For this review, use the dimensioned drawing (mm, ordinates from the lowest corner) and the shaded views. Give positions to 0.01 mm unless a question says otherwise; leave off trailing zeros. Loops run counter-clockwise (first coordinate to the right, second up) from the corner with the lowest first, then second, coordinate; pieces in that order, holes last. Notation, with made-up numbers: M -38.75,31 L -23.75,31 A22 cw -23.75,70 Z; hole C -20.5,53.25 d9. An arc over 180 degrees is marked long. Return JSON: item names as keys, results as strings.
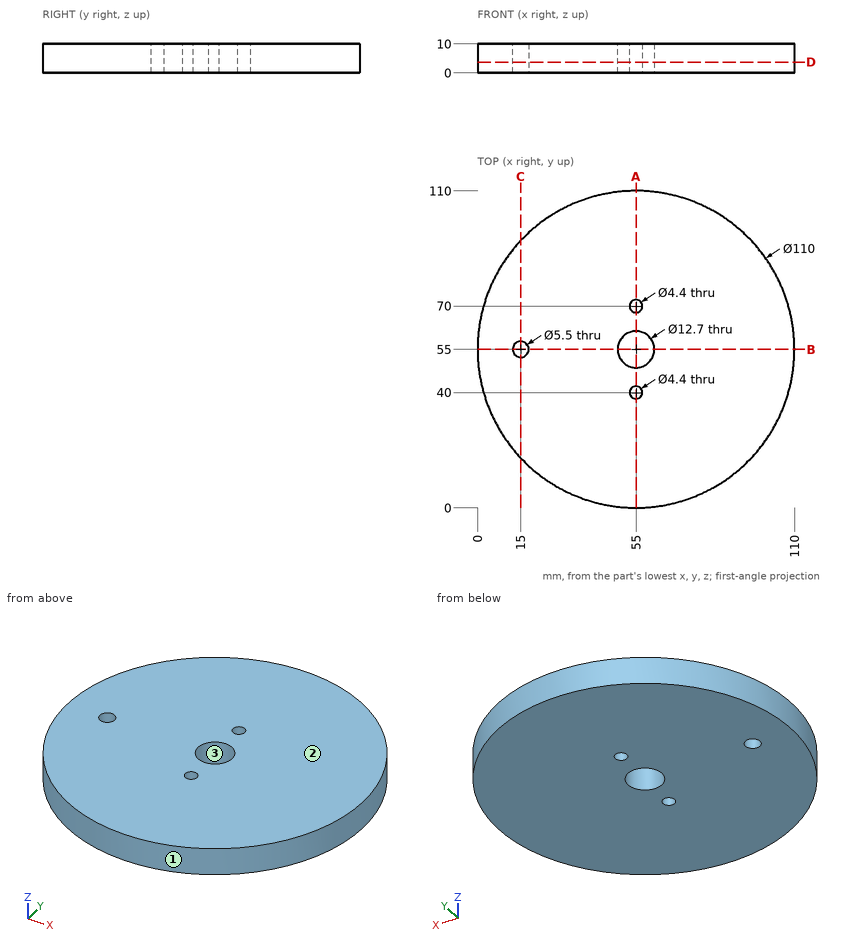
1) Insertion check: pin 1 (4 mm diameter, centred on y = 70, z = 5, fed in from +X); pin 2 (5 mm diameter, centred on x = 31.5, z = 7.5, fed in from +Y); pin 3 (5 mm diameter, centred on y = 27.5, z = 8.5, fed in from +X). Each pin has a flat end and moves straight along its axis. Give the tip position at first contact, or say it passes through.
From the geometry:
{"pin 1": "x = 108.44", "pin 2": "y = 105.83", "pin 3": "x = 103.99"}
2) The part is to be moulded in two halves that separate along X. For the marked faces 1, 2 and 3, say which applies: released by +X, released by -X, zero draft, split by the parting line, or undercut.
From the geometry:
{"face 1": "split by the parting line", "face 2": "zero draft", "face 3": "undercut"}
3) Consider section C-C on x = 15. Write out the cut boundary in (y, z).
From the geometry:
{"outline": "M 17.25,0 L 52.25,0 L 52.25,10 L 17.25,10 Z; M 57.75,0 L 92.75,0 L 92.75,10 L 57.75,10 Z"}
4) Consider section B-B on y = 55. Write out the cut boundary in (x, z), then the cut area to 3 significant figures.
From the geometry:
{"outline": "M 0,0 L 12.25,0 L 12.25,10 L 0,10 Z; M 17.75,0 L 48.65,0 L 48.65,10 L 17.75,10 Z; M 61.35,0 L 110,0 L 110,10 L 61.35,10 Z", "area": "918 mm²"}
5) Consider section D-D on z = 3.75. Write out the cut boundary in (x, y).
From the geometry:
{"outline": "C 55,55 d110; hole C 15,55 d5.5; hole C 55,55 d12.7; hole C 55,40 d4.4; hole C 55,70 d4.4"}
6) Consider section A-A on x = 55. Write out the cut boundary in (y, z), then the cut area to 3 significant figures.
From the geometry:
{"outline": "M 0,0 L 37.8,0 L 37.8,10 L 0,10 Z; M 42.2,0 L 48.65,0 L 48.65,10 L 42.2,10 Z; M 61.35,0 L 67.8,0 L 67.8,10 L 61.35,10 Z; M 72.2,0 L 110,0 L 110,10 L 72.2,10 Z", "area": "885 mm²"}
7) Wall thickness on L1, parallel to Y at x = 55, z = 3; L2, parallel to X at y = 53.5, z = 3.5; L3, parallel to X at y = 70, z = 8.25: over which ranges is each line inside the solid? List them lowest first. Write a range as from..to.
From the geometry:
{"L1": "0..37.8, 42.2..48.65, 61.35..67.8, 72.2..110", "L2": "0.02..12.7, 17.3..48.83, 61.17..109.98", "L3": "2.08..52.8, 57.2..107.92"}
